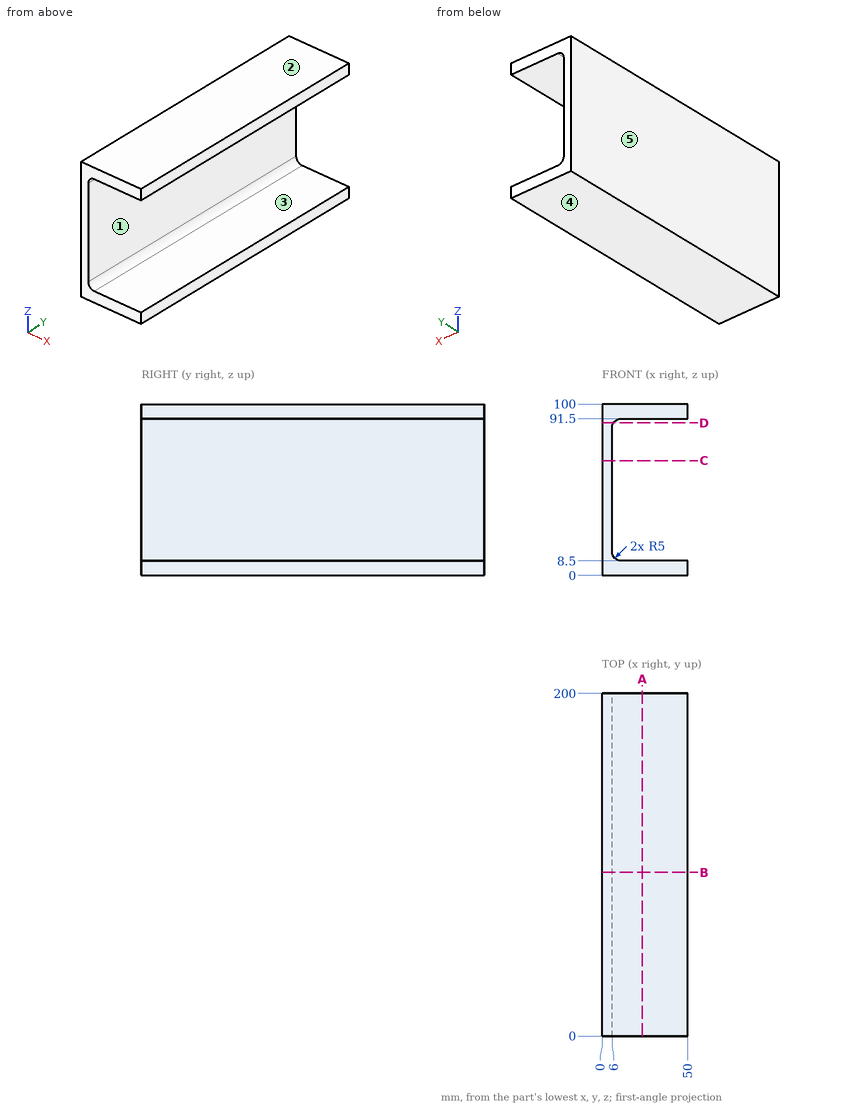
Geometry: see drawing. Coordinates: mm, zero at the bounding-box minimum. A direction names the side the tool comes from. Round coordinates to 2 decimals unless told otherwise and drop trailing zeros. Loops run counter-clockwise (first coordinate to the right, second up) from the corner with the lowest first, then second, coordinate; pieces in that order, holes last. Notation, with made-up numbers: (-1.75, 18) -> (42.25, 18) arc R23 cw to (42.25, 48) -> close; hole circle Ø4 at (83.5, -38). An arc over 180 degrees is marked (long way). Use one line per item in the form item = value. Start each with the question number.
Item 1: Section query B-B on y = 95.5. Return the cut outline in (x, z).
Item 2: Set-up query: the marked faces 1 and 2. Return all of +Z, -Z, +X, -X, +Y, -Y with unobstructed straight access to the full face (end or side cutting, diameter ignored); none if empty.
Item 3: Section query D-D on z = 89. Return the cut outline in (x, y).
Item 4: Material intervals for L1, parallel to Z at x = 19, y = 87; L2, parallel to X at y = 49.5, z = 35; L3, parallel to Z at x = 7, y = 167, sorted ascending. Write a range as from..to.
Item 5: Section query C-C on z = 67. Return the cut outline in (x, y).
Item 6: Contact query for a flat-ended pin moving along its axis: pin 1 Ø22 at (y, z) = (114, 57) entering from +X. Output: stop coordinate, or through.
Item 7: Section query A-A on x = 23.5. Return the cut outline in (y, z).
Item 8: Mould query, pull axis Z, two halves, no side actions, for the marked faces 3, 4 and 5. Classes: pulls with the +Z half, pulls with the -Z half, needs draft (parallel to the pull), parting line crosses it, or undercut.
Ans:
q1.outline = (0, 0) -> (50, 0) -> (50, 8.5) -> (11, 8.5) arc R5 cw to (6, 13.5) -> (6, 86.5) arc R5 cw to (11, 91.5) -> (50, 91.5) -> (50, 100) -> (0, 100) -> close
q2.face_1 = +X, +Y, -Y
q2.face_2 = +Z, +X, -X, +Y, -Y
q3.outline = (0, 0) -> (6.67, 0) -> (6.67, 200) -> (0, 200) -> close
q4.L1 = 0..8.5, 91.5..100
q4.L2 = 0..6
q4.L3 = 0..10.5, 89.5..100
q5.outline = (0, 0) -> (6, 0) -> (6, 200) -> (0, 200) -> close
q6.pin_1 = 6
q7.outline = (0, 0) -> (200, 0) -> (200, 8.5) -> (0, 8.5) -> close; (0, 91.5) -> (200, 91.5) -> (200, 100) -> (0, 100) -> close
q8.face_3 = undercut
q8.face_4 = pulls with the -Z half
q8.face_5 = needs draft
